Model file for the job. Use its own axes, mm. A direction names the side the tool comes from. Round coordinates to 2 decimals unless told otherwise and drop trailing zeros. Order: outer loops, then holes, each group sorted by start corner. A loop starts at its lowest first (then second) coordinate and runs counter-clockwise, first axis right, second up. Notation, with made-up numbers: (1, 48) -> (59, 48) arc R23 cw to (59, 79) -> close; hole circle Ø4 at (-30, 19). An arc over 180 degrees is marked (long way). Answer as CSV lines item,"result".
Autodesk Fusion 360 part; units mm, degrees
sketch "Sketch1" plane through (0, 0, 0) normal (0, 1, 0) x (1, 0, 0)
  circle A0 centre (0, 0) radius 73.5
  circle A1 centre (0, 0) radius 76.5
  dimension "d1" = 147
  dimension "d2" = 3
extrude "Extrude1" add sketch "Sketch1" along normal blind 2 makes body 1
ref_plane "WorkPlane1" through (0, -17, 0) normal (0, 1, 0) x (0, 0, 1)
sketch "Sketch2" plane through (0, -17, 0) normal (0, 1, 0) x (1, 0, 0)
  circle A0 centre (0, 0) radius 76.5
  circle A1 centre (0, 0) radius 76.51
  circle A2 centre (0, 0) radius 80.5
  dimension "d10" = 0.01
  dimension "d11" = 4
extrude "Extrude2" add sketch "Sketch2" along normal blind 2 separate body contours A2 makes body 2
ref_plane "WorkPlane2" through (0, 5, 0) normal (0, 1, 0) x (1, 0, 0)
sketch "Sketch3" plane through (0, 5, 0) normal (0, 1, 0) x (1, 0, 0)
  circle A0 centre (0, 0) radius 68.5
  circle A1 centre (0, 0) radius 73.5
  circle A2 centre (0, 0) radius 80.5
  dimension "d13" = 5
extrude "Extrude3" add sketch "Sketch3" against normal up to surface (3 mm away) contours A1 | A2 bodies 1
sketch "Sketch4" plane through (0, 2, 0) normal (0, -1, 0) x (1, 0, 0)
  circle A0 centre (0, 0) radius 80.5
  circle A1 centre (0, 0) radius 76.5
extrude "Extrude4" add sketch "Sketch4" along normal up to surface (17 mm away) bodies 1 2
sketch "Sketch5" plane through (0, -17, 0) normal (0, -1, 0) x (1, 0, 0)
  circle A0 centre (0, 0) radius 76.51
  circle A1 centre (0, 0) radius 80.5
  circle A2 centre (0, 0) radius 76.51
extrude "Extrude5" add sketch "Sketch5" along normal blind 3 bodies 1
sketch "Sketch6" plane through (0, 0, 0) normal (0, -1, 0) x (1, 0, 0)
  circle A0 centre (0, 0) radius 73.5
  circle A1 centre (0, 0) radius 76.5
extrude "Extrude6" add sketch "Sketch6" along normal blind 15 bodies 1
Q1. Saw through at C-C (y = -9.25). Write the cut outline in (x, z), plus the area to 3 significant figures.
Checks:
outline,"circle Ø161 at (0, 0); hole circle Ø147 at (0, 0)"
area,"3,390 mm²"
Q2. Saw through at A-A (x = 0). Write the cut outline in (y, z).
Checks:
outline,"(-20, -80.5) -> (5, -80.5) -> (5, -68.5) -> (2, -68.5) -> (2, -73.5) -> (-15, -73.5) -> (-15, -76.51) -> (-20, -76.51) -> close; (-20, 76.51) -> (-15, 76.51) -> (-15, 73.5) -> (2, 73.5) -> (2, 68.5) -> (5, 68.5) -> (5, 80.5) -> (-20, 80.5) -> close"
Q3. Flat gauge pins, fed straight in: pin 1 (6 mm diameter, centred on x = 50.5, y = -10.5, fed in from -Z); pin 2 (1 mm diameter, centred on y = -7.5, z = 46.5, fed in from -X); pin 3 (5 mm diameter, centred on x = -36.5, y = -13, fed in from -Z). Where does each tip first touch, or does it go through?
Checks:
pin 1,"z = -64.99"
pin 2,"x = -66.06"
pin 3,"z = -72.97"
Q4. Tool access for faces 1 (the cylindrical face through (-15.933, -6.381, 71.752)), 2 (the flat face through (71, -20, -29)): list every direction of +Z, -Z, +X, -X, +Y, -Y with a clear straight run to the whole face (end or side of a thin tool).
Checks:
face 1,"-Y"
face 2,"+Z, -Z, +X, -X, -Y"
Q5. Wall check: L1, parallel to Z at x = 0, y = -16.7; L2, parallel to X at y = -4.75, z = 0. Give the ranges that are in metal, low to high. Write a range as [from, to].
Checks:
L1,"[-80.5, -76.51], [76.51, 80.5]"
L2,"[-80.5, -73.5], [73.5, 80.5]"
Q6. Mould opens along Z. For faces 3 (the cylindrical face through (-80.422, -7.325, -3.539)), 4 (the cylindrical face through (65.337, 3.521, -20.576)), 5 (the flat face through (23, 5, -66)) say: +Z half, -Z half, draft (parallel to the pull), parting line (faces both ways), or undercut.
Checks:
face 3,"parting line"
face 4,"undercut"
face 5,"draft"
Q7. Saw through at B-B (z = 0). Write the cut outline in (x, y).
Checks:
outline,"(-80.5, -20) -> (-76.51, -20) -> (-76.51, -15) -> (-73.5, -15) -> (-73.5, 2) -> (-68.5, 2) -> (-68.5, 5) -> (-80.5, 5) -> close; (68.5, 2) -> (73.5, 2) -> (73.5, -15) -> (76.51, -15) -> (76.51, -20) -> (80.5, -20) -> (80.5, 5) -> (68.5, 5) -> close"
